```python
from build123d import *

# Parameters (mm, degrees)
F0_W     = 25.4
F0_H     = 25.4
F1_DEPTH = 22.225
F2_W     = 19.05
F2_H     = 19.05
F3_DEPTH = 15.875
F4_W     = 19.05
F4_H     = 19.05
F4_W_2   = 12.7
F4_H_2   = 12.7
F5_DEPTH = 6.35
F6_R     = 2.54


with BuildPart() as f1:
    # F0 (on Top) → F1 (new body)
    with BuildSketch(Plane.XY):
        with Locations((12.7, -12.7)):
            Rectangle(F0_W, F0_H)
    extrude(amount=F1_DEPTH)

    # F2 (on face) → F3 (cut)
    with BuildSketch(Plane(origin=(0, 0, 0), x_dir=(1, 0, 0), z_dir=(0, 0, -1))):
        with Locations((12.7, 12.7)):
            Rectangle(F2_W, F2_H)
    extrude(amount=-F3_DEPTH, mode=Mode.SUBTRACT)

    # F4 (on face) → F5 (join)
    with BuildSketch(Plane.XY.offset(22.225)):
        with Locations((12.7, -12.7)):
            Rectangle(F4_W, F4_H)
        with Locations((12.7, -12.7)):
            Rectangle(F4_W_2, F4_H_2, mode=Mode.SUBTRACT)
    extrude(amount=F5_DEPTH)

    # F6
    f6_edges = [f1.edges().sort_by_distance(p)[0] for p in [
        (0, 0, 11.1125),
        (0, -25.4, 11.1125),
        (25.4, 0, 11.1125),
        (3.175, -3.175, 25.4),
        (3.175, -22.225, 25.4),
        (22.225, -3.175, 25.4),
        (22.225, -22.225, 25.4),
        (25.4, -25.4, 11.1125),
    ]]
    fillet(f6_edges, radius=F6_R)


solid = f1.part
```
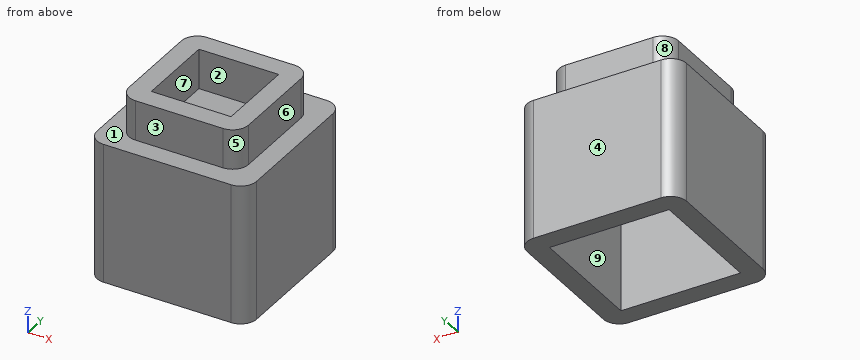
Here's how the part is built. I have some questions about the finished solid (model axes, mm). Face numbers are marked on the shaded views. A direction names the side the tool comes from. Round coordinates to 2 decimals unless told otherwise and drop trailing zeros. Order: outer loops, then holes, each group sorted by start corner. A loop starts at its lowest first (then second) coordinate and runs counter-clockwise, first axis right, second up. Notation, with made-up numbers: M 88.25,62 L 144.25,62 A22 cw 144.25,90 Z; hole C -29,19.5 d5. An arc over 180 degrees is marked long. Answer in a Markdown table with one row per item.
Item 1: Imagine slicing it at A-A, the plane z = 3.5. Write out the boundary of the cut face in (x, y) (3 decimals).
A:
| item | result |
|---|---|
| outline | M 0,-22.86 A2.54 ccw 2.54,-25.4 L 22.86,-25.4 A2.54 ccw 25.4,-22.86 L 25.4,-2.54 A2.54 ccw 22.86,0 L 2.54,0 A2.54 ccw 0,-2.54 Z; hole M 3.175,-22.225 L 22.225,-22.225 L 22.225,-3.175 L 3.175,-3.175 Z |
Item 2: If I drill on L1, parallel to X at y = -16, z = 7.5 (3 decimals); L2, parallel to Y at x = 9.75, z = 13.5 (3 decimals); L3, parallel to Z at x = 21.5, y = -19.25 (3 decimals), over which ranges is the centre line in solid material (lowest first)? Write a range as from..to.
A:
| item | result |
|---|---|
| L1 | x = 0..3.175, 22.225..25.4 |
| L2 | y = -25.4..-22.225, -3.175..0 |
| L3 | z = 15.875..28.575 |
Item 3: For the marked faces 5, 6, 7, 8 and 9, which set-ups out of +Z, -Z, +X, -X, +Y, -Y let a thin tool reach every point of the face, with its end or its side?
A:
| item | result |
|---|---|
| face 5 | +Z, +X, -Y |
| face 6 | +Z, +X, +Y, -Y |
| face 7 | +Z |
| face 8 | +Z, -X, +Y |
| face 9 | -Z |
Item 4: Imagine slicing it at C-C, the plane x = 7.5. Write out the boundary of the cut face in (y, z) (3 decimals).
A:
| item | result |
|---|---|
| outline | M -25.4,0 L -22.225,0 L -22.225,15.875 L -3.175,15.875 L -3.175,0 L 0,0 L 0,22.225 L -3.175,22.225 L -3.175,28.575 L -6.35,28.575 L -6.35,22.225 L -19.05,22.225 L -19.05,28.575 L -22.225,28.575 L -22.225,22.225 L -25.4,22.225 Z |
Item 5: I'm going to push flat-ended pins straight in: pin 1 (1 mm diameter, centred on x = 19, z = 25.5, fed in from +Y) (3 decimals); pin 2 (5 mm diameter, centred on y = -22, z = 24, fed in from -X); pin 3 (9.5 mm diameter, centred on x = 8.5, y = -15, fed in from -Z) (3 decimals); pin 4 (3 mm diameter, centred on x = 10, y = -9, fed in from +Z) (3 decimals). Where does each tip first touch, or does it pass through?
A:
| item | result |
|---|---|
| pin 1 | stops at y = -3.175 |
| pin 2 | stops at x = 0 |
| pin 3 | stops at z = 15.875 |
| pin 4 | stops at z = 22.225 |
Item 6: Imagine slicing it at D-D, the plane x = 23.5. Write out the boundary of the cut face in (y, z) (3 decimals), and give its area (3 significant figures).
A:
| item | result |
|---|---|
| outline | M -25.318,0 L -0.082,0 L -0.082,22.225 L -25.318,22.225 Z |
| area | 561 mm2 |
Item 7: Imagine slicing it at B-B, the plane y = -11.5. Write out the boundary of the cut face in (x, z) (3 decimals).
A:
| item | result |
|---|---|
| outline | M 0,0 L 3.175,0 L 3.175,15.875 L 22.225,15.875 L 22.225,0 L 25.4,0 L 25.4,22.225 L 22.225,22.225 L 22.225,28.575 L 19.05,28.575 L 19.05,22.225 L 6.35,22.225 L 6.35,28.575 L 3.175,28.575 L 3.175,22.225 L 0,22.225 Z |
Item 8: Thinking about a two-plate mould opening in Y: for the marked faces 1, 2, 3 and 4, which applies, +Y half, -Y half, draft (parallel to the pull), parting line (faces both ways), or undercut?
A:
| item | result |
|---|---|
| face 1 | draft |
| face 2 | undercut |
| face 3 | -Y half |
| face 4 | +Y half |
